from build123d import *

# Parameters (mm, degrees)
EXTRUDE_1_DEPTH     = 5.5
SKETCH_2_W          = 5.5
SKETCH_2_H          = 10
CUT_EXTRUDE_1_DEPTH = 126.901747406
SKETCH_5_W          = 5.5
SKETCH_5_H          = 5.5
CUT_EXTRUDE_2_DEPTH = 126.901747406


with BuildPart() as part:
    # ｽｹｯﾁ1 → ﾎﾞｽ - 押し出し1 (new body)
    with BuildSketch(Plane.XY):
        with BuildLine():
            Line((-10, -21.817424229), (-10, -125))
            Line((-10, -125), (10, -125))
            Line((10, -125), (10, -21.817424229))
            ThreePointArc((10, -21.817424229), (11.012114986, -21.324477099), (12, -20.784609691))
            ThreePointArc((12, -20.784609691), (13.464101615, -15.320508076), (8, -13.856406461))
            ThreePointArc((8, -13.856406461), (0, -16), (-8, -13.856406461))
            ThreePointArc((-8, -13.856406461), (-13.464101615, -15.320508076), (-12, -20.784609691))
            ThreePointArc((-12, -20.784609691), (-11.012114986, -21.324477099), (-10, -21.817424229))
        make_face()
    extrude(amount=EXTRUDE_1_DEPTH)

    # ｽｹｯﾁ2 → ｶｯﾄ - 押し出し1 (cut, through all)
    with BuildSketch(Plane.XY.offset(5.5)):
        with Locations((-7.25, -90)):
            Rectangle(SKETCH_2_W, SKETCH_2_H)
        with Locations((-7.25, -110)):
            Rectangle(SKETCH_2_W, SKETCH_2_H)
        with Locations((-7.25, -70)):
            Rectangle(SKETCH_2_W, SKETCH_2_H)
        with Locations((-7.25, -50)):
            Rectangle(SKETCH_2_W, SKETCH_2_H)
        with Locations((-7.25, -30)):
            Rectangle(SKETCH_2_W, SKETCH_2_H)
        with Locations((7.25, -110)):
            Rectangle(SKETCH_2_W, SKETCH_2_H)
        with Locations((7.25, -90)):
            Rectangle(SKETCH_2_W, SKETCH_2_H)
        with Locations((7.25, -70)):
            Rectangle(SKETCH_2_W, SKETCH_2_H)
        with Locations((7.25, -50)):
            Rectangle(SKETCH_2_W, SKETCH_2_H)
        with Locations((7.25, -30)):
            Rectangle(SKETCH_2_W, SKETCH_2_H)
    extrude(amount=-CUT_EXTRUDE_1_DEPTH, mode=Mode.SUBTRACT)

    # ｽｹｯﾁ5 → ｶｯﾄ - 押し出し2 (cut, through all)
    with BuildSketch(Plane.XY.offset(5.5)):
        with Locations((0, -40)):
            Rectangle(SKETCH_5_W, SKETCH_5_H)
        with Locations((0, -50)):
            Rectangle(SKETCH_5_W, SKETCH_5_H)
    extrude(amount=-CUT_EXTRUDE_2_DEPTH, mode=Mode.SUBTRACT)


solid = part.part
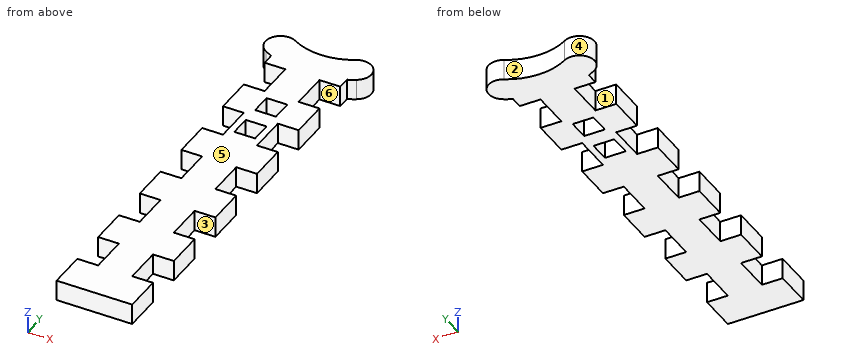
Design review of the part built by this model. Coordinates are the model's own, in mm. Face numbers are marked on the shaded views. A direction names the side the tool comes from. Round coordinates to 2 decimals unless told otherwise and drop trailing zeros. Write each loop counter-clockwise with the first axis right and the second up, starting at its lowest first coordinate (ties: lowest second). Pieces come first, ordered by that corner, then holes.
Item 1: Consider section C-C on y = -86. Give the boundary of the cut face in (x, z).
Item 2: Consider section B-B on z = 3.5. Count the separate pieces of the cut face and the enclosed holes in it, and give its area (3 significant figures).
Item 3: Consider section A-A on x = 5.5. Give the boundary of the cut face in (y, z).
Item 4: Wall thickness on L1, parallel to Y at x = -0.25, z = 1.2; L2, parallel to Y at x = -7.75, z = 1.6; L3, parallel to Y at x = -8.5, z = 4.4: over which ranges is each line inside the solid? List them lowest first.
Item 5: Draft analysis for pull direction Y (two halves, no side actions). For the marked faces 4, 5 and 6, state which applies: released by +Y, released by -Y, zero draft, split by the parting line, or undercut.
Item 6: For the marked faces 1, 2 and 3, list the 3-axis set-ups (+Z, -Z, +X, -X, +Y, -Y) from which the entire face can be reached by the end or side of a thin tool; tool diameter is ignored.
Item 7: For pin 1 Ø3 at (x, z) = (-7.5, 3.5) entering from +Y; pin 2 Ø3 at (y, z) = (-60, 3) entering from +X; pin 3 Ø1.6 at (y, z) = (-72.5, 4) entering from +X, all flat-tipped, find the tip position at first contact; note any pin that passes through.
Check values:
1. outline: (-4.5, 0) - (4.5, 0) - (4.5, 5.5) - (-4.5, 5.5) - close
2. separate pieces: 1
2. enclosed holes: 2
2. area: 1,640 mm2
3. outline: (-125, 0) - (-115, 0) - (-115, 5.5) - (-125, 5.5) - close; (-105, 0) - (-95, 0) - (-95, 5.5) - (-105, 5.5) - close; (-85, 0) - (-75, 0) - (-75, 5.5) - (-85, 5.5) - close; (-65, 0) - (-55, 0) - (-55, 5.5) - (-65, 5.5) - close; (-45, 0) - (-35, 0) - (-35, 5.5) - (-45, 5.5) - close; (-25, 0) - (-15.02, 0) - (-15.02, 5.5) - (-25, 5.5) - close
4. L1: y = -125 to -52.75, -47.25 to -42.75, -37.25 to -16
4. L2: y = -125 to -115, -105 to -95, -85 to -75, -65 to -55, -45 to -35, -25 to -14
4. L3: y = -125 to -115, -105 to -95, -85 to -75, -65 to -55, -45 to -35, -25 to -13.61
5. face 4: split by the parting line
5. face 5: zero draft
5. face 6: undercut
6. face 1: +Z, -Z, -X
6. face 2: +Z, -Z, +Y
6. face 3: +Z, -Z, +X
7. pin 1: stops at y = -13.45
7. pin 2: stops at x = 10
7. pin 3: stops at x = 4.5
